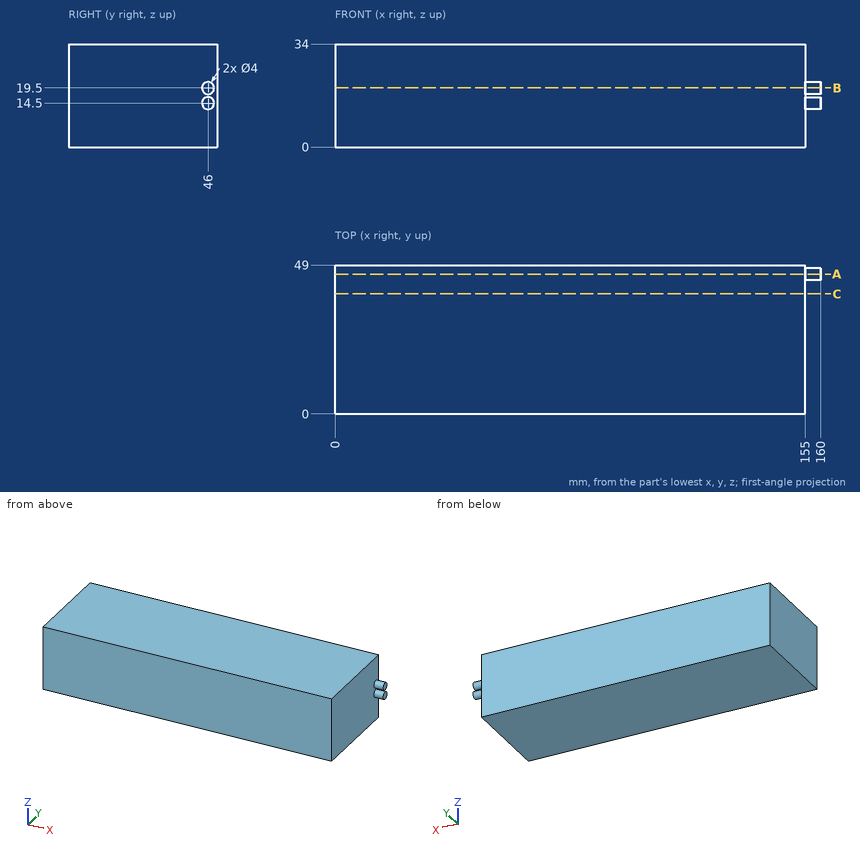
Here's the drawing with two shaded views (mm, measured from the low corner). I have some questions. Coordinates: 2 decimals unless noted, no trailing zeros. Order: outer loops, then holes, each group sorted by start corner. A loop starts at its lowest first (then second) coordinate and runs counter-clockwise, first axis right, second up. Notation, with made-up numbers: (-25, 13) - (-4, 13) arc R18 cw to (-4, 39) - close; hole circle Ø5 at (9, 86.25). An arc over 180 degrees is marked (long way). Use CSV: the item, a comma, the result in double quotes. Start each with the question number.
1. Suppose I cut it at C-C on y = 39.5. List the corners of the cut face in (x, z) for me, then the cut area to 3 significant figures.
2. Please list where this line runs through material, in increasing order: line 1 (X direction, y = 32.5, z = 25). Write a range as from..to.
3. Suppose I cut it at B-B on z = 19.5. List the corners of the cut face in (x, y) for me.
4. I'm going to push a flat-ended pin straight in: pin 1 (10 mm diameter, centred on y = 24.5, z = 14, fed in from +X). Where does the tip first touch, or does it pass through?
5. Suppose I cut it at A-A on y = 46. List the corners of the cut face in (x, z) for me, then the cut area to 3 significant figures.
Output:
1,outline,"(0, 0) - (155, 0) - (155, 34) - (0, 34) - close"
1,area,"5,270 mm2"
2,line 1,"x = 0..155"
3,outline,"(0, 0) - (155, 0) - (155, 44) - (160, 44) - (160, 48) - (155, 48) - (155, 49) - (0, 49) - close"
4,pin 1,"stops at x = 155"
5,outline,"(0, 0) - (155, 0) - (155, 12.5) - (160, 12.5) - (160, 16.5) - (155, 16.5) - (155, 17.5) - (160, 17.5) - (160, 21.5) - (155, 21.5) - (155, 34) - (0, 34) - close"
5,area,"5,310 mm2"
